Verification items for the finished model (mm, model axes). Give positions to 0.01 mm unless a question says otherwise; leave off trailing zeros. Order: outer loops, then holes, each group sorted by start corner. A loop starts at its lowest first (then second) coordinate and runs counter-clockwise, first axis right, second up. Notation, with made-up numbers: (61.25, -14.75) - (66.25, -14.75) arc R22 ccw to (66.25, -1.75) - close; hole circle Ø8 at (49, 71.5). An arc over 180 degrees is marked (long way). Answer as a JSON object with one key per item and string values. Group by question number.
(1) Depth check by flat-ended pin: pin 1 Ø3 at (x, y) = (44.5, 0) entering from -Z; pin 2 Ø0.9 at (y, z) = (-5, 2) entering from +X; pin 3 Ø0.9 at (y, z) = (-6, 2) entering from -X; pin 4 Ø0.9 at (x, z) = (120, 2) entering from -Y. Enter the tip coordinate at first touch or a pass-through.
(2) Section check A-A (z = 2.05). Count the separate pieces of the cut face and the enclosed holes in it, then the cut area to 3 significant figures.
(3) Thickness scan on line 1 (X direction, y = -8, z = 1.8); line 2 (X direction, y = -6.5, z = 0.35); line 3 (X direction, y = -5, z = 1.95). Record the ranges inside material, lowest first.
(4) Section check B-B (x = 101.5). Record the boundary of the cut face in (y, z).
```python
from build123d import *

# Parameters (mm, degrees)
F0_W     = 259.72
F0_H     = 6.4
F1_DEPTH = 3
F3_DEPTH = 3
F4_R     = 2.63999
F5_R     = 1.75
F5_W     = 17.25
F5_H     = 2.2
F6_DEPTH = 3.001
F7_W     = 31.12
F7_H     = 2
F8_DEPTH = 3.001


# Not quite as in the source:
# - a fillet or chamfer is up to 0.001 mm smaller than in the source, because OpenCascade refuses the exact size
# - ends of sketch curves that miss each other by under 0.0002 mm in the source are joined


with BuildPart() as f1:
    # F0 (on Top) → F1 (new body)
    with BuildSketch(Plane.XY):
        Rectangle(F0_W, F0_H)
    extrude(amount=F1_DEPTH)

    # F2 (on Top) → F3 (join)
    with BuildSketch(Plane.XY):
        with BuildLine():
            Line((129.86, -10.59), (129.86, -3.2))
            Line((129.86, -3.2), (124.58, -3.2))
            Line((124.58, -3.2), (124.58, -7.95))
            Line((124.58, -7.95), (125.47, -7.95))
            ThreePointArc((125.47, -7.95), (127.22, -6.2), (128.97, -7.95))
            ThreePointArc((128.97, -7.95), (128.4574368671, -9.1874368671), (127.22, -9.7))
            Line((127.22, -9.7), (127.22, -10.59))
            Line((127.22, -10.59), (129.86, -10.59))
        make_face()
        with BuildLine():
            Line((125.47, -7.95), (124.58, -7.95))
            Line((124.58, -7.95), (124.58, -10.59))
            Line((124.58, -10.59), (127.22, -10.59))
            Line((127.22, -10.59), (127.22, -9.7))
            ThreePointArc((127.22, -9.7), (125.9825631329, -9.1874368671), (125.47, -7.95))
        make_face()
        Polygon((53.66, -10.59), (53.66, -3.2), (48.38, -3.2), (48.38, -7.95), (48.38, -10.59), align=None)
        with BuildLine():
            ThreePointArc((52.77, -7.95), (51.02, -9.7), (49.27, -7.95))
            ThreePointArc((49.27, -7.95), (51.02, -6.2), (52.77, -7.95))
        make_face(mode=Mode.SUBTRACT)
        Polygon((-22.54, -3.2), (-27.82, -3.2), (-27.82, -7.95), (-27.82, -10.59), (-22.54, -10.59), align=None)
        with BuildLine():
            ThreePointArc((-23.43, -7.95), (-25.18, -9.7), (-26.93, -7.95))
            ThreePointArc((-26.93, -7.95), (-25.18, -6.2), (-23.43, -7.95))
        make_face(mode=Mode.SUBTRACT)
    extrude(amount=F3_DEPTH)

    # F4 (radius 2.64 in the source; OpenCascade refuses exactly that, so slightly less here)
    f4_edges = [f1.edges().sort_by_distance(p)[0] for p in [
        (48.38, -10.59, 1.5),
        (53.66, -10.59, 1.5),
        (124.58, -10.59, 1.5),
        (129.86, -10.59, 1.5),
        (-27.82, -10.59, 1.5),
        (-22.54, -10.59, 1.5),
    ]]
    fillet(f4_edges, radius=F4_R)

    # F5 (on face) → F6 (cut, through all)
    with BuildSketch(Plane.XY.offset(3)):
        with BuildLine():
            Line((124.58, 3.2), (124.58, 1))
            Line((124.58, 1), (124.58, -1))
            Line((124.58, -1), (124.58, -3.2))
            Line((124.58, -3.2), (124.58, -7.95001))
            ThreePointArc((124.58, -7.95001), (125.3532351687, -9.8167648313), (127.21999, -10.59))
            ThreePointArc((127.21999, -10.59), (129.0867648313, -9.8167648313), (129.86, -7.95001))
            Line((129.86, -7.95001), (129.86, 3.2))
            Line((129.86, 3.2), (124.58, 3.2))
        make_face()
        with Locations((127.22, -7.95)):
            Circle(F5_R, mode=Mode.SUBTRACT)
        with Locations((115.955, 2.1)):
            Rectangle(F5_W, F5_H)
        with Locations((115.955, -2.1)):
            Rectangle(F5_W, F5_H)
    extrude(amount=-F6_DEPTH, mode=Mode.SUBTRACT)

    # F7 (on face) → F8 (cut, through all)
    with BuildSketch(Plane.XY.offset(3)):
        Polygon((-129.86, 3.2), (-129.86, 1), (-98.74, 1), (-81.49, 1), (-81.49, 3.2), align=None)
        Polygon((-129.86, -1), (-129.86, -3.2), (-81.49, -3.2), (-81.49, -1), (-98.74, -1), align=None)
        with Locations((-114.3, 0)):
            Rectangle(F7_W, F7_H)
    extrude(amount=-F8_DEPTH, mode=Mode.SUBTRACT)


solid = f1.part
```
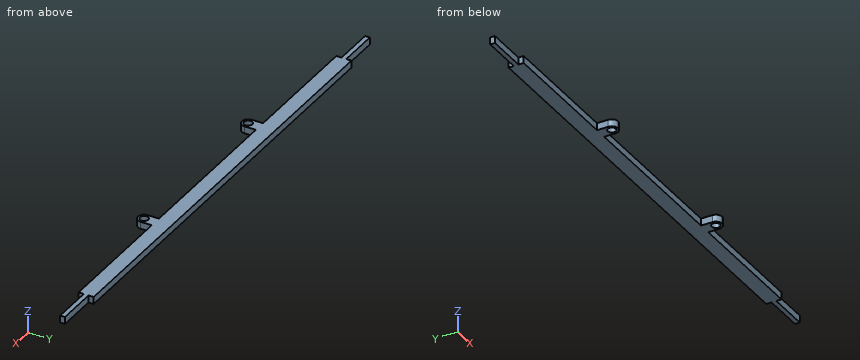
Solutions:
{
 "1": {"pin 1": "stops at z = 0", "pin 2": "stops at x = 53.66", "pin 3": "stops at x = -27.82", "pin 4": "stops at y = -1"},
 "2": {"separate pieces": "1", "enclosed holes": "2", "area": "1,330 mm2"},
 "3": {"line 1": "x = -27.82 to -26.93, -23.43 to -22.54, 48.38 to 49.27, 52.77 to 53.66", "line 2": "x = -27.82 to -26.16, -24.2 to -22.54, 48.38 to 50.04, 52 to 53.66", "line 3": "x = -27.82 to -22.54, 48.38 to 53.66"},
 "4": {"outline": "(-3.2, 0) - (3.2, 0) - (3.2, 3) - (-3.2, 3) - close"}
}
